Could you check a few things on this model? Use its own coordinates, in mm. A direction names the side the tool comes from. Coordinates: 2 decimals unless noted, no trailing zeros. Write each loop counter-clockwise with the first axis right and the second up, starting at its lowest first coordinate (ties: lowest second). Pieces come first, ordered by that corner, then holes. Notation, with made-up numbers: M -36,-5 L 5,-5 A27 ccw 5,33 Z; hole C -5,29 d4. An arc over 180 degrees is marked long. Answer as CSV lines item,"result". Start each with the question number.
Item 1: On a 3-axis mill with a long thin cutter (end or side, diameter ignored), from which of +Z, -Z, +X, -X, +Y, -Y can I reach the whole of each face in a straight line? I mean faces 5 (the flat face through (-3, -75.095, -3)), 6 (the flat face through (-41.275, -94, -3)), 7 (the flat face through (-3, -151.295, -3)), 8 (the flat face through (-14.287, -72, -3)). Say none if no direction works.
Item 2: If I drill on line 1 along Y through (x, z) = (-41.5, -4); line 2 along Y through (x, z) = (-30, -3.75); line 3 along X through (y, z) = (-141.5, -5.25) (3 decimals), over which ranges is the centre line in solid material (lowest first)? Write a range as [from, to].
Item 3: Suppose I cut it at B-B, the plane x = -32. Write out the boundary of the cut face in (y, z).
Item 4: We'd pull the mould along X, two halves only. Please class faces 1 (the flat face through (-26.988, -167, -3)), 2 (the flat face through (-44, -100.495, -3)), 3 (the flat face through (-47.625, -82, -3)), 4 (the flat face through (-33.338, -72, -3)): +X half, -X half, draft (parallel to the pull), parting line (faces both ways), or undercut.
Item 5: I'm going to push flat-ended pins straight in: P1, Ø1.9, axis at y = -72, z = -2, coming from the -X side (3 decimals); P2, Ø1.9, axis at x = -3.5, z = -2.5, coming from the -Y side; P3, Ø1.9, axis at x = -3.5, z = -2, coming from the +Y side. Where does each tip first touch, or does it pass through?
Item 6: Suppose I cut it at A-A, the plane x = -3. Write out the boundary of the cut face in (y, z).
Item 7: Suppose I cut it at C-C, the plane y = -144.5. Write out the boundary of the cut face in (x, z) (3 decimals), and give its area (3 significant figures).
```python
from build123d import *

# Parameters (mm, degrees)
SKETCH1_W           = 47.625
SKETCH1_H           = 101.6
BOSS_EXTRUDE1_DEPTH = 6.35
SKETCH4_W           = 12.7
SKETCH4_H           = 12.7
CUT_EXTRUDE1_DEPTH  = 177.991271514
LPATTERN1_COUNT     = 3
LPATTERN1_PITCH     = 25.4
LPATTERN1_COL_COUNT = 3
LPATTERN1_COL_PITCH = 25.4
SKETCH3_W           = 6.35
SKETCH3_H           = 12.7
CUT_EXTRUDE2_DEPTH  = 177.991271514


with BuildPart() as part:
    # Sketch1 → Boss-Extrude1 (new body)
    with BuildSketch(Plane.XY):
        with Locations((-23.8125, -119.54508231)):
            Rectangle(SKETCH1_W, SKETCH1_H)
    extrude(amount=-BOSS_EXTRUDE1_DEPTH)

    # Sketch4 → Cut-Extrude1 (cut, through all)
    with BuildSketch(Plane.XY):
        with Locations((0, -119.54508231)):
            Rectangle(SKETCH4_W, SKETCH4_H)
        with Locations((-47.625, -119.54508231)):
            Rectangle(SKETCH4_W, SKETCH4_H)
    cut_extrude1 = extrude(amount=-CUT_EXTRUDE1_DEPTH, mode=Mode.SUBTRACT)

    # LPattern1: Cut-Extrude1 ×3
    with Locations(*[(0, -i * LPATTERN1_PITCH, 0) for i in range(1, LPATTERN1_COUNT)]):
        add(cut_extrude1, mode=Mode.SUBTRACT)

    # LPattern1 col: Cut-Extrude1 ×3
    with Locations(*[(0, i * LPATTERN1_COL_PITCH, 0) for i in range(1, LPATTERN1_COL_COUNT)]):
        add(cut_extrude1, mode=Mode.SUBTRACT)

    # Sketch3 → Cut-Extrude2 (cut, through all)
    with BuildSketch(Plane.XY):
        with Locations((-17.4625, -68.74508231)):
            Rectangle(SKETCH3_W, SKETCH3_H)
        with Locations((-30.1625, -68.74508231)):
            Rectangle(SKETCH3_W, SKETCH3_H)
        with Locations((-30.1625, -170.34508231)):
            Rectangle(SKETCH3_W, SKETCH3_H)
        with Locations((-17.4625, -170.34508231)):
            Rectangle(SKETCH3_W, SKETCH3_H)
    extrude(amount=-CUT_EXTRUDE2_DEPTH, mode=Mode.SUBTRACT)


solid = part.part
```
Ans:
1,face 5,"+Z, -Z, +X, +Y"
1,face 6,"+Z, -Z, -X"
1,face 7,"+Z, -Z, +X"
1,face 8,"+Z, -Z, +Y"
2,line 1,"y = [-164, -151.3], [-138.6, -125.9], [-113.2, -100.5], [-87.8, -75.1]"
2,line 2,"y = [-164, -75.1]"
2,line 3,"x = [-41.275, -6.35]"
3,outline,"M -164,-6.35 L -75.1,-6.35 L -75.1,0 L -164,0 Z"
4,face 1,"undercut"
4,face 2,"draft"
4,face 3,"-X half"
4,face 4,"undercut"
5,P1,"stops at x = -41.275"
5,P2,"stops at y = -164"
5,P3,"stops at y = -75.1"
6,outline,"M -164,-6.35 L -151.3,-6.35 L -151.3,0 L -164,0 Z; M -138.6,-6.35 L -125.9,-6.35 L -125.9,0 L -138.6,0 Z; M -113.2,-6.35 L -100.5,-6.35 L -100.5,0 L -113.2,0 Z; M -87.8,-6.35 L -75.1,-6.35 L -75.1,0 L -87.8,0 Z"
7,outline,"M -41.275,-6.35 L -6.35,-6.35 L -6.35,0 L -41.275,0 Z"
7,area,"222 mm^2"
